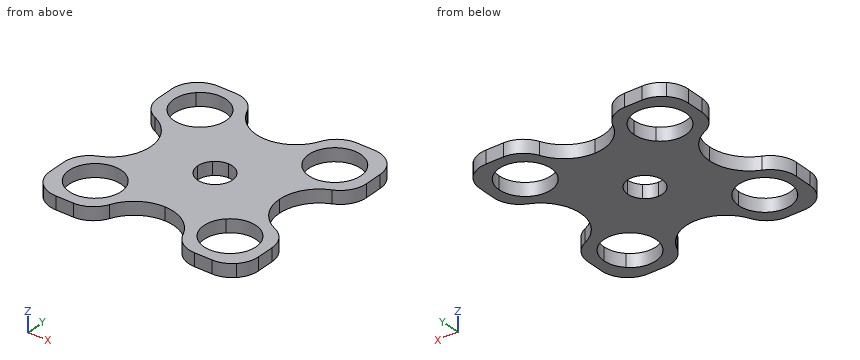
from build123d import *

# Parameters (mm, degrees)
F1_DEPTH = 4.7625
F2_R     = 9.525


with BuildPart() as f1:
    # F0 (on Top) → F1 (new body)
    with BuildSketch(Plane.XY):
        with BuildLine():
            Line((-17.8944237276, -17.8944237276), (-4.4901280605, -4.4901280605))
            ThreePointArc((-4.4901280605, -4.4901280605), (-5.8666350314, -2.4300397955), (-6.35, 0))
            Line((-6.35, 0), (-23.4970493061, 0))
            ThreePointArc((-23.4970493061, 0), (-27.774154539, -10.325845461), (-38.1, -14.6029506939))
            Line((-38.1, -14.6029506939), (-38.1, -28.575))
            ThreePointArc((-38.1, -28.575), (-37.3749525472, -32.2200596933), (-35.3101920908, -35.3101920908))
            Line((-35.3101920908, -35.3101920908), (-31.3648079092, -31.3648079092))
            ThreePointArc((-31.3648079092, -31.3648079092), (-31.3648079092, -17.8944237276), (-17.8944237276, -17.8944237276))
        make_face()
        with BuildLine():
            ThreePointArc((-6.35, 0), (-5.8666350314, 2.4300397955), (-4.4901280605, 4.4901280605))
            Line((-4.4901280605, 4.4901280605), (-17.8944237276, 17.8944237276))
            ThreePointArc((-17.8944237276, 17.8944237276), (-31.3648079092, 17.8944237276), (-31.3648079092, 31.3648079092))
            Line((-31.3648079092, 31.3648079092), (-35.3101920908, 35.3101920908))
            ThreePointArc((-35.3101920908, 35.3101920908), (-37.3749525472, 32.2200596933), (-38.1, 28.575))
            Line((-38.1, 28.575), (-38.1, 14.6029506939))
            ThreePointArc((-38.1, 14.6029506939), (-27.774154539, 10.325845461), (-23.4970493061, 0))
            Line((-23.4970493061, 0), (-6.35, 0))
        make_face()
        with BuildLine():
            ThreePointArc((-4.4901280605, 4.4901280605), (-2.4300397955, 5.8666350314), (0, 6.35))
            Line((0, 6.35), (0, 23.4970493061))
            ThreePointArc((0, 23.4970493061), (-10.325845461, 27.774154539), (-14.6029506939, 38.1))
            Line((-14.6029506939, 38.1), (-28.575, 38.1))
            ThreePointArc((-28.575, 38.1), (-32.2200596933, 37.3749525472), (-35.3101920908, 35.3101920908))
            Line((-35.3101920908, 35.3101920908), (-31.3648079092, 31.3648079092))
            ThreePointArc((-31.3648079092, 31.3648079092), (-20.9845561251, 33.4295683656), (-15.1046158184, 24.6296158184))
            ThreePointArc((-15.1046158184, 24.6296158184), (-15.8296632712, 20.9845561251), (-17.8944237276, 17.8944237276))
            Line((-17.8944237276, 17.8944237276), (-4.4901280605, 4.4901280605))
        make_face()
        with BuildLine():
            ThreePointArc((0, 6.35), (2.4300397955, 5.8666350314), (4.4901280605, 4.4901280605))
            Line((4.4901280605, 4.4901280605), (17.8944237276, 17.8944237276))
            ThreePointArc((17.8944237276, 17.8944237276), (17.8944237276, 31.3648079092), (31.3648079092, 31.3648079092))
            Line((31.3648079092, 31.3648079092), (35.3101920908, 35.3101920908))
            ThreePointArc((35.3101920908, 35.3101920908), (32.2200596933, 37.3749525472), (28.575, 38.1))
            Line((28.575, 38.1), (14.6029506939, 38.1))
            ThreePointArc((14.6029506939, 38.1), (10.325845461, 27.774154539), (0, 23.4970493061))
            Line((0, 23.4970493061), (0, 6.35))
        make_face()
        with BuildLine():
            ThreePointArc((4.4901280605, 4.4901280605), (5.8666350314, 2.4300397955), (6.35, 0))
            Line((6.35, 0), (23.4970493061, 0))
            ThreePointArc((23.4970493061, 0), (27.774154539, 10.325845461), (38.1, 14.6029506939))
            Line((38.1, 14.6029506939), (38.1, 28.575))
            ThreePointArc((38.1, 28.575), (37.3749525472, 32.2200596933), (35.3101920908, 35.3101920908))
            Line((35.3101920908, 35.3101920908), (31.3648079092, 31.3648079092))
            ThreePointArc((31.3648079092, 31.3648079092), (33.4295683656, 28.2746755117), (34.1546158184, 24.6296158184))
            ThreePointArc((34.1546158184, 24.6296158184), (28.2746755117, 15.8296632712), (17.8944237276, 17.8944237276))
            Line((17.8944237276, 17.8944237276), (4.4901280605, 4.4901280605))
        make_face()
        with BuildLine():
            Line((23.4970493061, 0), (6.35, 0))
            ThreePointArc((6.35, 0), (5.8666350314, -2.4300397955), (4.4901280605, -4.4901280605))
            Line((4.4901280605, -4.4901280605), (17.8944237276, -17.8944237276))
            ThreePointArc((17.8944237276, -17.8944237276), (28.2746755117, -15.8296632712), (34.1546158184, -24.6296158184))
            ThreePointArc((34.1546158184, -24.6296158184), (33.4295683656, -28.2746755117), (31.3648079092, -31.3648079092))
            Line((31.3648079092, -31.3648079092), (35.3101920908, -35.3101920908))
            ThreePointArc((35.3101920908, -35.3101920908), (37.3749525472, -32.2200596933), (38.1, -28.575))
            Line((38.1, -28.575), (38.1, -14.6029506939))
            ThreePointArc((38.1, -14.6029506939), (27.774154539, -10.325845461), (23.4970493061, 0))
        make_face()
        with BuildLine():
            Line((17.8944237276, -17.8944237276), (4.4901280605, -4.4901280605))
            ThreePointArc((4.4901280605, -4.4901280605), (2.4300397955, -5.8666350314), (0, -6.35))
            Line((0, -6.35), (0, -23.4970493061))
            ThreePointArc((0, -23.4970493061), (10.325845461, -27.774154539), (14.6029506939, -38.1))
            Line((14.6029506939, -38.1), (28.575, -38.1))
            ThreePointArc((28.575, -38.1), (32.2200596933, -37.3749525472), (35.3101920908, -35.3101920908))
            Line((35.3101920908, -35.3101920908), (31.3648079092, -31.3648079092))
            ThreePointArc((31.3648079092, -31.3648079092), (17.8944237276, -31.3648079092), (17.8944237276, -17.8944237276))
        make_face()
        with BuildLine():
            Line((0, -23.4970493061), (0, -6.35))
            ThreePointArc((0, -6.35), (-2.4300397955, -5.8666350314), (-4.4901280605, -4.4901280605))
            Line((-4.4901280605, -4.4901280605), (-17.8944237276, -17.8944237276))
            ThreePointArc((-17.8944237276, -17.8944237276), (-15.8296632712, -20.9845561251), (-15.1046158184, -24.6296158184))
            ThreePointArc((-15.1046158184, -24.6296158184), (-20.9845561251, -33.4295683656), (-31.3648079092, -31.3648079092))
            Line((-31.3648079092, -31.3648079092), (-35.3101920908, -35.3101920908))
            ThreePointArc((-35.3101920908, -35.3101920908), (-32.2200596933, -37.3749525472), (-28.575, -38.1))
            Line((-28.575, -38.1), (-14.6029506939, -38.1))
            ThreePointArc((-14.6029506939, -38.1), (-10.325845461, -27.774154539), (0, -23.4970493061))
        make_face()
    extrude(amount=F1_DEPTH)

    # F2
    f2_edges = [f1.edges().sort_by_distance(p)[0] for p in [
        (-38.1, 14.602951, 2.38125),
        (-38.1, -14.602951, 2.38125),
        (-14.602951, -38.1, 2.38125),
        (14.602951, -38.1, 2.38125),
        (38.1, -14.602951, 2.38125),
        (38.1, 14.602951, 2.38125),
        (-14.602951, 38.1, 2.38125),
        (14.602951, 38.1, 2.38125),
    ]]
    fillet(f2_edges, radius=F2_R)


solid = f1.part
Check sheet for the modelled part. Datum: model origin and axes. Units: mm. Round coordinates to 2 decimals unless told otherwise and drop trailing zeros. Order: outer loops, then holes, each group sorted by start corner. A loop starts at its lowest first (then second) coordinate and runs counter-clockwise, first axis right, second up.
Q1. Depth check by flat-ended pin: P1, Ø2, axis at x = -12.5, z = 4, coming from the +Y side; P2, Ø6, axis at x = -25, y = 8.5, coming from the -Z side. Enter the tip coordinate at first touch or a pass-through.
Filled sheet:
P1: stops at y = 32.52
P2: stops at z = 0
Q2. Cross-section at D-D, the plane x = -21. Enter the section's corners in (y, z).
Filled sheet:
outline: (-38.03, 0) - (-33.44, 0) - (-33.44, 4.76) - (-38.03, 4.76) - close; (-15.82, 0) - (15.82, 0) - (15.82, 4.76) - (-15.82, 4.76) - close; (33.44, 0) - (38.03, 0) - (38.03, 4.76) - (33.44, 4.76) - close
Q3. Scan lines: L1, parallel to X at y = 20.5, z = 3.4; L2, parallel to Y at x = -31.5, z = 2.9; L3, parallel to X at y = 30, z = 1.55. Record each from-to range of solid material in increasing order.
Filled sheet:
L1: x = -37.95 to -33.21, -16.05 to 16.05, 33.21 to 37.95
L2: y = -37.64 to -31.23, -18.03 to -13.03, 13.03 to 18.03, 31.23 to 37.64
L3: x = -37.99 to -32.5, -16.76 to -12.15, 12.15 to 16.76, 32.5 to 37.99
Q4. Cross-section at C-C, the plane z = 2.3. Give the number of separate pieces and of enclosed holes in the cut face, plus the area to 3 significant figures.
Filled sheet:
separate pieces: 1
enclosed holes: 5
area: 3,050 mm2
Q5. Cross-section at B-B, the plane y = -26.5. Enter the section's corners in (x, z).
Filled sheet:
outline: (-38.1, 0) - (-33.97, 0) - (-33.97, 4.76) - (-38.1, 4.76) - close; (-15.29, 0) - (-8.87, 0) - (-8.87, 4.76) - (-15.29, 4.76) - close; (8.87, 0) - (15.29, 0) - (15.29, 4.76) - (8.87, 4.76) - close; (33.97, 0) - (38.1, 0) - (38.1, 4.76) - (33.97, 4.76) - close
Q6. Cross-section at A-A, the plane x = 3.5. Enter the section's corners in (y, z), plus the area to 3 significant figures.
Filled sheet:
outline: (-23.92, 0) - (-5.3, 0) - (-5.3, 4.76) - (-23.92, 4.76) - close; (5.3, 0) - (23.92, 0) - (23.92, 4.76) - (5.3, 4.76) - close
area: 177 mm2
